CAD build for the part. Positions are in the model's coordinates, mm. A direction names the side the tool comes from. Give positions to 0.01 mm unless a question says otherwise; leave off trailing zeros. Write each loop counter-clockwise with the first axis right and the second up, starting at its lowest first coordinate (ties: lowest second). Pieces come first, ordered by that corner, then holes. Notation, with made-up numbers: (-10, 6) - (0, 6) arc R33 ccw to (0, 43) - close; hole circle Ø5 at (50, 17.5). An arc over 180 degrees is marked (long way). Answer as a JSON object with one key per item and string values.
from build123d import *

# Parameters (mm, degrees)
SCHIZZO1_W                   = 60
SCHIZZO1_H                   = 30
ESTRUSIONE_ESTRUSIONE1_DEPTH = 5
SCHIZZO2_W                   = 60
SCHIZZO2_H                   = 8
ESTRUSIONE_ESTRUSIONE2_DEPTH = 20
SCHIZZO3_R                   = 5
TAGLIO_ESTRUSIONE1_DEPTH     = 8
RACCORDO1_R                  = 20
SCHIZZO4_W                   = 60
SCHIZZO4_H                   = 15
ESTRUSIONE_ESTRUSIONE3_DEPTH = 10
SCHIZZO6_R                   = 8
TAGLIO_ESTRUSIONE2_DEPTH     = 15
SCHIZZO8_W                   = 60
SCHIZZO8_H                   = 4.7
ESTRUSIONE_ESTRUSIONE4_DEPTH = 10
SCHIZZO9_R                   = 6.3
TAGLIO_ESTRUSIONE3_DEPTH     = 5
SCHIZZO10_R                  = 2
TAGLIO_ESTRUSIONE4_DEPTH     = 37.742346142
SCHIZZO11_W                  = 60
SCHIZZO11_H                  = 8
TAGLIO_ESTRUSIONE5_DEPTH     = 25
SCHIZZO14_W                  = 60
SCHIZZO14_H                  = 5
TAGLIO_ESTRUSIONE7_DEPTH     = 7
SCHIZZO12_R                  = 2
ESTRUSIONE_ESTRUSIONE5_DEPTH = 4
SCHIZZO17_W                  = 60
SCHIZZO17_H                  = 15
TAGLIO_ESTRUSIONE9_DEPTH     = 3
TAGLIO_ESTRUSIONE10_REACH    = 38.058
TAGLIO_ESTRUSIONE12_DEPTH    = 8
RACCORDO2_R                  = 5
RACCORDO3_R                  = 10


with BuildPart() as part:
    # Schizzo1 → Estrusione-Estrusione1 (new body)
    with BuildSketch(Plane.XY):
        Rectangle(SCHIZZO1_W, SCHIZZO1_H)
    extrude(amount=ESTRUSIONE_ESTRUSIONE1_DEPTH)

    # Schizzo2 → Estrusione-Estrusione2 (add)
    with BuildSketch(Plane.XY.offset(5)):
        with Locations((0, 11)):
            Rectangle(SCHIZZO2_W, SCHIZZO2_H)
    extrude(amount=ESTRUSIONE_ESTRUSIONE2_DEPTH)

    # Schizzo3 → Taglio-Estrusione1 (cut)
    with BuildSketch(Plane(origin=(0, 15, 0), x_dir=(1, 0, 0), z_dir=(0, 1, 0))):
        with Locations(Location((11, -13, 0), (0, 0, 270))):
            Circle(SCHIZZO3_R)
        with Locations(Location((-11, -13, 0), (0, 0, 270))):
            Circle(SCHIZZO3_R)
    extrude(amount=-TAGLIO_ESTRUSIONE1_DEPTH, mode=Mode.SUBTRACT)

    # Raccordo1
    raccordo1_edges = [part.edges().sort_by_distance(p)[0] for p in [
        (30, 11, 25),
        (-30, 11, 25),
    ]]
    fillet(raccordo1_edges, radius=RACCORDO1_R)

    # Schizzo4 → Estrusione-Estrusione3 (add)
    with BuildSketch(Plane.XY.offset(5)):
        with Locations((0, -0.5)):
            Rectangle(SCHIZZO4_W, SCHIZZO4_H)
    extrude(amount=ESTRUSIONE_ESTRUSIONE3_DEPTH)

    # Schizzo6 → Taglio-Estrusione2 (cut)
    with BuildSketch(Plane.XZ.offset(8)):
        with Locations((0, 13)):
            Circle(SCHIZZO6_R)
    extrude(amount=-TAGLIO_ESTRUSIONE2_DEPTH, mode=Mode.SUBTRACT)

    # Schizzo8 → Estrusione-Estrusione4 (add)
    with BuildSketch(Plane.XY.offset(15)):
        with Locations((0, -0.85)):
            Rectangle(SCHIZZO8_W, SCHIZZO8_H)
    extrude(amount=-ESTRUSIONE_ESTRUSIONE4_DEPTH)

    # Schizzo9 → Taglio-Estrusione3 (cut)
    with BuildSketch(Plane.XZ.offset(3.2)):
        with Locations((0, 13)):
            Circle(SCHIZZO9_R)
    extrude(amount=-TAGLIO_ESTRUSIONE3_DEPTH, mode=Mode.SUBTRACT)

    # Schizzo10 → Taglio-Estrusione4 (cut, through all)
    with BuildSketch(Plane.XY.offset(15)):
        with Locations((12, -0.85)):
            Circle(SCHIZZO10_R)
        with Locations((-12, -0.85)):
            Circle(SCHIZZO10_R)
    extrude(amount=-TAGLIO_ESTRUSIONE4_DEPTH, mode=Mode.SUBTRACT)

    # Schizzo11 → Taglio-Estrusione5 (cut)
    with BuildSketch(Plane(origin=(0, 0, 0), x_dir=(-1, 0, 0), z_dir=(0, 0, -1))):
        with Locations((0, 11)):
            Rectangle(SCHIZZO11_W, SCHIZZO11_H)
    extrude(amount=-TAGLIO_ESTRUSIONE5_DEPTH, mode=Mode.SUBTRACT)

    # Schizzo14 → Taglio-Estrusione7 (cut)
    with BuildSketch(Plane.XZ.offset(15)):
        with Locations((0, 2.5)):
            Rectangle(SCHIZZO14_W, SCHIZZO14_H)
    extrude(amount=-TAGLIO_ESTRUSIONE7_DEPTH, mode=Mode.SUBTRACT)

    # Schizzo12 → Estrusione-Estrusione5 (add)
    with BuildSketch(Plane.XY):
        with BuildLine():
            Line((-8, -8.006435696), (8, -8.006435696))
            Line((8, -8.006435696), (20, -8.006435696))
            Line((20, -8.006435696), (20, -12.006435696))
            ThreePointArc((20, -12.006435696), (24, -16.006435696), (28, -12.006435696))
            Line((28, -12.006435696), (28, -5.256435696))
            Line((28, -5.256435696), (-28, -5.256435696))
            Line((-28, -5.256435696), (-28, -12.006435696))
            ThreePointArc((-28, -12.006435696), (-24, -16.006435696), (-20, -12.006435696))
            Line((-20, -12.006435696), (-20, -8.006435696))
            Line((-20, -8.006435696), (-8, -8.006435696))
        make_face()
        with Locations((24, -12.006435696)):
            Circle(SCHIZZO12_R, mode=Mode.SUBTRACT)
        with Locations(Location((-24, -12.006435696, 0), (0, 0, 180))):
            Circle(SCHIZZO12_R, mode=Mode.SUBTRACT)
    extrude(amount=ESTRUSIONE_ESTRUSIONE5_DEPTH)

    # Schizzo17 → Taglio-Estrusione9 (cut)
    with BuildSketch(Plane.XY.offset(15)):
        with Locations((0, -0.5)):
            Rectangle(SCHIZZO17_W, SCHIZZO17_H)
    extrude(amount=-TAGLIO_ESTRUSIONE9_DEPTH, mode=Mode.SUBTRACT)

    # Taglio-Estrusione10: up to this face of the body (flat: up to its plane)
    taglio_estrusione10_end = Plane(part.part.faces().sort_by_distance((-18.942934314, -0.495179718, 12))[0])
    # Schizzo18 → Taglio-Estrusione10 (cut, up to the picked face)
    with BuildSketch(Plane(origin=(0, 0, 0), x_dir=(-1, 0, 0), z_dir=(0, 0, -1)), mode=Mode.PRIVATE) as taglio_estrusione10_sk1:
        with BuildLine():
            Line((-26, -8.043105695), (-26, -12.006435696))
            Line((-26, -12.006435696), (-22, -12.006435696))
            Line((-22, -12.006435696), (-22, -8.043105695))
            ThreePointArc((-22, -8.043105695), (-24, -6.043105695), (-26, -8.043105695))
        make_face()
    taglio_estrusione10_tool1 = split(extrude(taglio_estrusione10_sk1.sketch, amount=-TAGLIO_ESTRUSIONE10_REACH, mode=Mode.PRIVATE), bisect_by=taglio_estrusione10_end, keep=Keep.BOTH, mode=Mode.PRIVATE)
    # Schizzo18 → Taglio-Estrusione10 (cut, up to the picked face)
    with BuildSketch(Plane(origin=(0, 0, 0), x_dir=(-1, 0, 0), z_dir=(0, 0, -1)), mode=Mode.PRIVATE) as taglio_estrusione10_sk2:
        with BuildLine():
            Line((22, -12.006435696), (22, -8.043105695))
            ThreePointArc((22, -8.043105695), (24, -6.043105695), (26, -8.043105695))
            Line((26, -8.043105695), (26, -12.006435696))
            Line((26, -12.006435696), (22, -12.006435696))
        make_face()
    taglio_estrusione10_tool2 = split(extrude(taglio_estrusione10_sk2.sketch, amount=-TAGLIO_ESTRUSIONE10_REACH, mode=Mode.PRIVATE), bisect_by=taglio_estrusione10_end, keep=Keep.BOTH, mode=Mode.PRIVATE)
    add(taglio_estrusione10_tool1.solids().sort_by(Axis((24, -9.221369, 0), (0, 0, 1)))[0], mode=Mode.SUBTRACT)
    add(taglio_estrusione10_tool2.solids().sort_by(Axis((-24, -9.221369, 0), (0, 0, 1)))[0], mode=Mode.SUBTRACT)

    # Schizzo20 → Taglio-Estrusione12 (cut)
    with BuildSketch(Plane.XY.offset(4)):
        Polygon((-27.25, -9.91949407), (-24, -11.795882445), (-20.75, -9.91949407), (-20.75, -6.166717321), (-24, -4.290328946), (-27.25, -6.166717321), align=None)
    taglio_estrusione12 = extrude(amount=TAGLIO_ESTRUSIONE12_DEPTH, mode=Mode.SUBTRACT)

    # Specchia1: Taglio-Estrusione12 across plane
    add(taglio_estrusione12.mirror(Plane(origin=(0, 0, 0), x_dir=(0, 0, 1), z_dir=(1, 0, 0))), mode=Mode.SUBTRACT)

    # Raccordo2
    # the kernel refuses this fillet: 5 mm, written as the material it adds along each edge
    with BuildSketch(Plane(origin=(28, -8, 4), x_dir=(1, 0, 0), z_dir=(0, 0, -1))) as raccordo2_piece_1:
        with BuildLine():
            CenterArc((5, 4), RACCORDO2_R, 180, 53.130102354)
            Line((0, 4), (0, 0))
            Line((0, 0), (2, 0))
        make_face()
    extrude(amount=4)
    with BuildSketch(Plane(origin=(-28, -8, 0), x_dir=(2.553025400590997e-07, -0.9999999999999674, 0), z_dir=(0, 0, 1))) as raccordo2_piece_2:
        with BuildLine():
            CenterArc((4.000000448, -4.999998721), RACCORDO2_R, 89.959025437, 53.171095231)
            Line((-5.11e-07, -2), (-0.400000606, -1.700000128))
            ThreePointArc((-0.400000606, -1.700000128), (-0.500000255, -0.999999872), (-0.5, 1.28e-07))
            Line((-0.5, 1.28e-07), (1.28e-07, 0.5))
            Line((1.28e-07, 0.5), (4.003933724, 0.499999872))
            Line((4.003933724, 0.499999872), (4.003576153, 0))
        make_face()
    extrude(amount=4)

    # Raccordo3
    raccordo3_edges = [part.edges().sort_by_distance(p)[0] for p in [
        (-20, -8.006435696, 2),
        (20, -8.006435696, 2),
    ]]
    fillet(raccordo3_edges, radius=RACCORDO3_R)


solid = part.part
Item 1: Probe line 1 (X direction, y = -6.75, z = 8.25); line 2 (Y direction, x = -12, z = 8.5); line 3 (X direction, y = -0.5, z = 7.75). List the from-to ranges inside material, lowest first. Write a range as from..to.
Entries:
{"line 1": "-30..-27.25, -20.75..-6.44, 6.44..20.75, 27.25..30", "line 2": "-8..-2.85, 1.15..7", "line 3": "-30..-13.97, -10.03..-3.48, 3.48..10.03, 13.97..30"}
Item 2: Cut at C-C (z = 2). State how many separate pieces and enclosed holes the cut face has, and give its area (3 significant figures).
Entries:
{"separate pieces": "1", "enclosed holes": "4", "area": "963 mm2"}
Item 3: Cut at A-A (y = -0.85). Give the cut face in (x, z).
Entries:
{"outline": "(-30, 0) - (-14, 0) - (-14, 12) - (-30, 12) - close; (-10, 0) - (10, 0) - (10, 12) - (6.22, 12) arc R6.3 cw to (-6.22, 12) - (-10, 12) - close; (14, 0) - (30, 0) - (30, 12) - (14, 12) - close"}
Item 4: Flat gauge pins, fed straight in: P1, Ø1.4, axis at x = 28, z = 8, coming from the -Y side; P2, Ø2, axis at y = -11, z = 3, coming from the +X side; P3, Ø4, axis at x = -2.5, y = -9.5, coming from the -Z side; P4, Ø4.5, axis at y = -10.5, z = 1, coming from the -X side. Where does each tip first touch, or does it go through?
Entries:
{"P1": "y = -8", "P2": "x = 28.42", "P3": "z = 0", "P4": "x = -29.69"}
Item 5: Mould opens along Y. For faces 1 (the flat face through (0, -2, 0)), 2 (the flat face through (29, -8, 8)), 3 (the cylindrical face through (-23.956, -6.044, 1.972)) say: +Y half, -Y half, draft (parallel to the pull), parting line (faces both ways), or undercut.
Entries:
{"face 1": "draft", "face 2": "-Y half", "face 3": "undercut"}
Item 6: Cut at B-B (z = 10.25). Give the cut face in (x, y).
Entries:
{"outline": "(-30, -8) - (-27.25, -8) - (-27.25, -6.17) - (-24, -4.29) - (-20.75, -6.17) - (-20.75, -8) - (-7.51, -8) - (-7.51, -3.2) - (-5.67, -3.2) - (-5.67, 1.5) - (-7.51, 1.5) - (-7.51, 7) - (-30, 7) - close; (5.67, -3.2) - (7.51, -3.2) - (7.51, -8) - (20.75, -8) - (20.75, -6.17) - (24, -4.29) - (27.25, -6.17) - (27.25, -8) - (30, -8) - (30, 7) - (7.51, 7) - (7.51, 1.5) - (5.67, 1.5) - close; hole circle Ø4 at (-12, -0.85); hole circle Ø4 at (12, -0.85)"}
Item 7: Which spindle directions (+Z, -Z, +X, -X, +Y, -Y) get a long thin tool onto all of the face, cutting with end or side? Do faces 4 (the cylindrical face through (-28.515, -9.791, 1.972)), 5 (the flat face through (27.25, -7, 8)), 6 (the cylindrical face through (-24.044, -14.006, 1.972)), 7 (the flat face through (0, 1.5, 6)). Say none if no direction does.
Entries:
{"face 4": "+Z, -Z, -X, -Y", "face 5": "+Z, -Y", "face 6": "+Z, -Z", "face 7": "+Z, +Y"}
